Here's how the part is built. I have some questions about the finished solid (model axes, mm). A direction names the side the tool comes from. Round coordinates to 2 decimals unless told otherwise and drop trailing zeros. Loops run counter-clockwise (first coordinate to the right, second up) from the corner with the lowest first, then second, coordinate; pieces in that order, holes last. Notation, with made-up numbers: M 38,-32 L 88,-32 A21 cw 88,-14 Z; hole C 60,57 d7. An arc over 180 degrees is marked long. Use a Markdown table: item, result.
Autodesk Inventor part; units mm, degrees
ref_plane "YZ Plane" through (0, 0, 0) normal (1, 0, 0) x (0, 1, 0)
ref_plane "XZ Plane" through (0, 0, 0) normal (0, 1, 0) x (-1, 0, 0)
ref_plane "XY Plane" through (0, 0, 0) normal (0, 0, 1) x (1, 0, 0)
sketch "Sketch1" plane through (0, 0, 0) normal (0, 1, 0) x (-1, 0, 0)
  line L0 (50, 50) -> (-50, 50)
  line L1 (-50, 50) -> (-50, -50)
  line L2 (-50, -50) -> (50, -50)
  line L3 (50, -50) -> (50, 50)
  point P0 (0, 0)
  point P1 (50, 0)
  point P2 (0, 50)
  dimension "d0" = 100
  dimension "d1" = 100
extrude "Extrusion1" add sketch "Sketch1" along normal blind 50
sketch "Sketch2" plane through (0, 50, 0) normal (0, 1, 0) x (1, 0, 0)
  line L0 (50, -50) -> (50, 50) construction
  line L1 (50, 50) -> (-50, 50) construction
  line L2 (-50, 50) -> (-50, -50) construction
  line L3 (-50, -50) -> (50, -50) construction
  line L4 (-50, 50) -> (-50, -50) construction
  line L5 (-50, 0) -> (50, 0) construction
  line L6 (50, -50) -> (50, 50) construction
  arc A0 (40, 0) -> (-40, 0) centre (0, 0) ccw
  line L7 (-40, 0) -> (40, 0) construction
  line L8 (-40, 0) -> (40, 0)
  dimension "d4" = 80
revolve "Revolution1" cut sketch "Sketch2" angle 360 about axis through (-50, 50, 0) along (1, 0, 0)
sketch "Sketch3" plane through (0, 50, 0) normal (0, 1, 0) x (1, 0, 0)
  circle A0 centre (0, 0) radius 40 construction
  line L0 (50, -50) -> (50, 50) construction
  line L1 (50, 50) -> (-50, 50) construction
  line L2 (-50, 50) -> (-50, -50) construction
  line L3 (-50, -50) -> (50, -50) construction
  circle A1 centre (-38, 38) radius 5
  line L4 (50, 50) -> (-50, 50) construction
  line L5 (0, 50) -> (0, 0) construction
  line L6 (0, 0) -> (50, 0) construction
  line L7 (50, -50) -> (50, 50) construction
  dimension "d6" = 10
  dimension "d7" = 12
  dimension "d8" = 12
extrude "Extrusion2" cut sketch "Sketch3" against normal blind 50
pattern_linear "Rectangular Pattern1" count 2 spacing 78 along (1, 0, 0) count 2 spacing 78 along (0, 0, 1) of "Extrusion2"
sketch "Sketch4" plane through (50, 0, 50) normal (1, 0, 0) x (0, 0, -1)
  line L0 (0, 0) -> (100, 0) construction
  line L1 (100, 0) -> (100, 50) construction
  line L2 (0, 50) -> (100, 50) construction
  line L3 (0, 0) -> (0, 50) construction
  arc A0 (43, 50) -> (57, 50) centre (50, 50) ccw
  line L4 (57, 50) -> (43, 50)
  line L5 (0, 50) -> (100, 50)
  point P0 (50, 0)
  dimension "d17" = 7
extrude "Extrusion3" cut sketch "Sketch4" against normal up to surface
fillet "Fillet1" radius 5 4 edges at (-50, 25, 50) (50, 25, 50) (50, 25, -50) (-50, 25, -50)
properties part number "molde1-01"
Q1. I need wall thicknesses on line 1 (X direction, y = 15.5, z = -38); line 2 (Z direction, x = -40, y = 8.5). Which ranges of each line are inside material? Lowest first, please. Write a range as from..to.
Return value:
| item | result |
|---|---|
| line 1 | x = -50..-43, -33..35, 45..50 |
| line 2 | z = -50..-42.58, -33.42..35.42, 44.58..50 |
Q2. Imagine slicing it at B-B, the plane x = -38. Please give me the cut outline in (y, z), then the cut area to 3 significant figures.
Return value:
| item | result |
|---|---|
| outline | M 0,-50 L 50,-50 L 50,-43 L 0,-43 Z; M 0,-33 L 50,-33 L 50,-12.49 A12.49 cw 50,12.49 L 50,35 L 0,35 Z; M 0,45 L 50,45 L 50,50 L 0,50 Z |
| area | 3,750 mm^2 |
Q3. For faces 5 (the cylindrical face through (45, 43, 0)), 6 (the cylindrical face through (35, 25, 40)), which set-ups out of +Z, -Z, +X, -X, +Y, -Y let a thin tool reach every point of the face, with its end or its side?
Return value:
| item | result |
|---|---|
| face 5 | +X, +Y |
| face 6 | +Y, -Y |
Q4. Imagine slicing it at D-D, the plane z = 0. Please give me the cut outline in (x, y), then the cut area to 3 significant figures.
Return value:
| item | result |
|---|---|
| outline | M -50,0 L 50,0 L 50,43 L 39.38,43 A40 cw -40,50 L -50,50 Z |
| area | 2,420 mm^2 |
Q5. Imagine slicing it at C-C, the plane y = 21.5. Please give me the cut outline in (x, z).
Return value:
| item | result |
|---|---|
| outline | M -50,-45 A5 ccw -45,-50 L 45,-50 A5 ccw 50,-45 L 50,45 A5 ccw 45,50 L -45,50 A5 ccw -50,45 Z; hole C -38,-38 d10; hole C -38,40 d10; hole C 0,0 d56.13; hole C 40,-38 d10; hole C 40,40 d10 |
Q6. Imagine slicing it at A-A, the plane z = -38. Please give me the cut outline in (x, y).
Return value:
| item | result |
|---|---|
| outline | M -50,0 L -43,0 L -43,50 L -50,50 Z; M -33,0 L 35,0 L 35,50 L 12.49,50 A12.49 cw -12.49,50 L -33,50 Z; M 45,0 L 50,0 L 50,50 L 45,50 Z |
Q7. We'd pull the mould along X, two halves only. Please class faces 1 (the flat face through (50, 25, 1)), 2 (the cylindrical face through (36, 25, -41)), 3 (the cylindrical face through (-43, 25, 40)), 4 (the flat face through (-1, 25, 50)): pulls with the +X half, pulls with the -X half, needs draft (parallel to the pull), parting line crosses it, or undercut.
Return value:
| item | result |
|---|---|
| face 1 | pulls with the +X half |
| face 2 | undercut |
| face 3 | undercut |
| face 4 | needs draft |
Q8. Will these pins go through, and if not, where does the flat tip stop? P1, Ø16, axis at x = -38, z = -38, coming from the -Y side; P2, Ø8, axis at x = 40, z = 40, coming from the +Y side.
Return value:
| item | result |
|---|---|
| P1 | stops at y = 0 |
| P2 | passes through |
